Model file for the job. Use its own axes, mm. A direction names the side the tool comes from. Give positions to 0.01 mm unless a question says otherwise; leave off trailing zeros. Write each loop counter-clockwise with the first axis right and the second up, starting at its lowest first coordinate (ties: lowest second). Pieces come first, ordered by that corner, then holes. Notation, with made-up numbers: (79, 29.25) - (136, 29.25) arc R10 cw to (136, 44.25) - close; hole circle Ø6 at (7, 46). An arc over 180 degrees is marked (long way). Use CSV: the item, a comma, the result in double quotes.
from build123d import *

# Parameters (mm, degrees)
SKETCH1_W                 = 32.4
SKETCH1_H                 = 32.4
BOSS_EXTRUDE1_DEPTH       = 98.5
SKETCH2_R                 = 11.65
CUT_EXTRUDE1_DEPTH        = 88.5
SKETCH3_R                 = 6.5
CUT_EXTRUDE2_DEPTH        = 99.398410022
F_1_0MM_DOWEL_HOLE1_D     = 2.8
F_1_0MM_DOWEL_HOLE1_DEPTH = 7
F_1_0MM_DOWEL_HOLE1_TIP   = 0.841204867
SKETCH7_R                 = 2.5
CUT_EXTRUDE3_DEPTH        = 14
SKETCH8_W                 = 6.5
SKETCH8_H                 = 98.5
BOSS_EXTRUDE2_DEPTH       = 8.64
SKETCH14_W                = 30.956114244
SKETCH14_H                = 32.4
CUT_EXTRUDE6_DEPTH        = 50
SKETCH11_W                = 20.4
SKETCH11_H                = 31.75
CUT_EXTRUDE4_DEPTH        = 107.197037106
SKETCH12_W                = 20.4
SKETCH12_H                = 31.75
CUT_EXTRUDE5_DEPTH        = 15
SKETCH23_W                = 8.64
SKETCH23_H                = 6.5
BOSS_EXTRUDE3_DEPTH       = 11.5
F_1_0MM_DOWEL_HOLE3_D     = 2.8
F_1_0MM_DOWEL_HOLE3_DEPTH = 5
F_1_0MM_DOWEL_HOLE3_TIP   = 0.841204867


with BuildPart() as part:
    # Sketch1 → Boss-Extrude1 (new body)
    with BuildSketch(Plane(origin=(0, 0, 0), x_dir=(1, 0, 0), z_dir=(0, 1, 0))):
        with Locations((-6.730344165, -20.189509634)):
            Rectangle(SKETCH1_W, SKETCH1_H)
        Polygon((11.469655835, -27.889509634), (9.469655835, -29.389509634), (9.469655835, -31.389509634), (11.469655835, -32.889509634), align=None)
        Polygon((11.469655835, -7.489509634), (9.469655835, -8.989509634), (9.469655835, -10.989509634), (11.469655835, -12.489509634), align=None)
    extrude(amount=BOSS_EXTRUDE1_DEPTH)

    # Sketch2 → Cut-Extrude1 (cut)
    with BuildSketch(Plane(origin=(0, 98.5, 0), x_dir=(1, 0, 0), z_dir=(0, 1, 0))):
        with Locations(Location((-6.730344165, -20.189509634, 0), (0, 0, 270))):
            Circle(SKETCH2_R)
    extrude(amount=-CUT_EXTRUDE1_DEPTH, mode=Mode.SUBTRACT)

    # Sketch3 → Cut-Extrude2 (cut, through all)
    with BuildSketch(Plane(origin=(0, 10, 0), x_dir=(1, 0, 0), z_dir=(0, 1, 0))):
        with Locations(Location((-6.730344165, -20.189509634, 0), (0, 0, 270))):
            Circle(SKETCH3_R)
    extrude(amount=-CUT_EXTRUDE2_DEPTH, mode=Mode.SUBTRACT)

    # Ø1.0mm Dowel Hole1
    with Locations(Plane(origin=(0, 98.5, 0), x_dir=(1, 0, 0), z_dir=(0, 1, 0))):
        with Locations((-18.730344165, -8.189509634), (5.269655835, -8.189509634), (5.269655835, -32.189509634), (-18.730344165, -32.189509634)):
            Hole(F_1_0MM_DOWEL_HOLE1_D / 2, depth=F_1_0MM_DOWEL_HOLE1_DEPTH)
            with Locations((0, 0, -(F_1_0MM_DOWEL_HOLE1_DEPTH + F_1_0MM_DOWEL_HOLE1_TIP / 2))):  # 118° drill point
                Cone(0, F_1_0MM_DOWEL_HOLE1_D / 2, F_1_0MM_DOWEL_HOLE1_TIP, mode=Mode.SUBTRACT)

    # Sketch7 → Cut-Extrude3 (cut)
    with BuildSketch(Plane(origin=(0, 0, 3.989509634), x_dir=(-1, 0, 0), z_dir=(0, 0, -1))):
        with Locations((6.730344165, 4.5)):
            Circle(SKETCH7_R)
    extrude(amount=-CUT_EXTRUDE3_DEPTH, mode=Mode.SUBTRACT)

    # Sketch8 → Boss-Extrude2 (add)
    with BuildSketch(Plane(origin=(9.469655835, 0, 0), x_dir=(0, 0, -1), z_dir=(1, 0, 0))):
        with Locations((-20.189509634, 49.25)):
            Rectangle(SKETCH8_W, SKETCH8_H)
    extrude(amount=BOSS_EXTRUDE2_DEPTH)

    # Sketch14 → Cut-Extrude6 (cut)
    with BuildSketch(Plane.XZ):
        with Locations((24.947712957, 20.189509634)):
            Rectangle(SKETCH14_W, SKETCH14_H)
    extrude(amount=-CUT_EXTRUDE6_DEPTH, mode=Mode.SUBTRACT)

    # Sketch11 → Cut-Extrude4 (cut, through all)
    with BuildSketch(Plane.XY.offset(36.389509634)):
        with Locations((-6.730344165, 72.625)):
            Rectangle(SKETCH11_W, SKETCH11_H)
        with Locations((-6.730344165, 30.875)):
            Rectangle(SKETCH11_W, SKETCH11_H)
    extrude(amount=-CUT_EXTRUDE4_DEPTH, mode=Mode.SUBTRACT)

    # Sketch12 → Cut-Extrude5 (cut)
    with BuildSketch(Plane.ZY.offset(22.930344165)):
        with Locations((20.189509634, 72.625)):
            Rectangle(SKETCH12_W, SKETCH12_H)
        with Locations((20.189509634, 30.875)):
            Rectangle(SKETCH12_W, SKETCH12_H)
    extrude(amount=-CUT_EXTRUDE5_DEPTH, mode=Mode.SUBTRACT)

    # Sketch23 → Boss-Extrude3 (add)
    with BuildSketch(Plane(origin=(0, 98.5, 0), x_dir=(1, 0, 0), z_dir=(0, 1, 0))):
        with Locations((13.789655835, -20.189509634)):
            Rectangle(SKETCH23_W, SKETCH23_H)
    extrude(amount=BOSS_EXTRUDE3_DEPTH)

    # Ø1.0mm Dowel Hole3
    with Locations(Plane(origin=(18.109655835, 0, 0), x_dir=(0, 0, -1), z_dir=(1, 0, 0))):
        with Locations((-20.189509634, 105), (-20.189509634, 55), (-20.189509634, 65), (-20.189509634, 95)):
            Hole(F_1_0MM_DOWEL_HOLE3_D / 2, depth=F_1_0MM_DOWEL_HOLE3_DEPTH)
            with Locations((0, 0, -(F_1_0MM_DOWEL_HOLE3_DEPTH + F_1_0MM_DOWEL_HOLE3_TIP / 2))):  # 118° drill point
                Cone(0, F_1_0MM_DOWEL_HOLE3_D / 2, F_1_0MM_DOWEL_HOLE3_TIP, mode=Mode.SUBTRACT)


solid = part.part
(1) Wall check: probe 1 along Y at (x, z) = (-5, 33.5); probe 2 along Z at (x, y) = (-18, 34); probe 3 along Z at (x, y) = (15.4, 65). Give the ranges that are in metal, low to high. Write a range as [from, to].
Checked values:
probe 1,"y = [0, 15], [46.75, 56.75], [88.5, 98.5]"
probe 2,"z = [3.99, 9.99], [30.39, 36.39]"
probe 3,"z = [16.94, 18.79], [21.59, 23.44]"
(2) 3-axis set-ups, long thin cutter, end or side, ignore diameter. For faces 5 (the face through (4.89, 64.29, 21.04)), 6 (the face through (-19, 56.75, 20)), 7 (the face through (9.47, 104, 20)), 8 (the face through (-20, 72, 30.39)), 9 (the face through (-16.93, 72, 33)): which of +Z, -Z, +X, -X, +Y, -Y reach the whole face in a straight line?
Checked values:
face 5,"+Y"
face 6,"none"
face 7,"+Z, -Z, -X, +Y"
face 8,"-X"
face 9,"+Z, -Z"
(3) Saw through at D-D, the plane y = 4.5. List the corners of the cut face in (x, z).
Checked values:
outline,"(-22.93, 3.99) - (-9.23, 3.99) - (-9.23, 14.19) arc R6.5 cw (long way) to (-4.23, 14.19) - (-4.23, 3.99) - (9.47, 3.99) - (9.47, 36.39) - (-22.93, 36.39) - close"
(4) Pull direction Z, two halves, no side cores. Call faces 1 (the face through (5.573, 94.951, 33.556)), 2 (the face through (18.11, 80, 20)), 3 (the face through (-7, 49, 36.39)), 4 (the face through (5.49, 90.8, 32.28)): released by +Z, released by -Z, zero draft, split by the parting line, or undercut.
Checked values:
face 1,"undercut"
face 2,"zero draft"
face 3,"released by +Z"
face 4,"undercut"
(5) Saw through at A-A, the plane y = 45.5. List the corners of the cut face in (x, z).
Checked values:
outline,"(-22.93, 3.99) - (-16.93, 3.99) - (-16.93, 9.99) - (-22.93, 9.99) - close; (-22.93, 30.39) - (-16.93, 30.39) - (-16.93, 36.39) - (-22.93, 36.39) - close; (3.47, 3.99) - (9.47, 3.99) - (9.47, 36.39) - (3.47, 36.39) - (3.47, 25.82) arc R11.65 cw to (3.47, 14.56) - close"
(6) Flat gauge pins, fed straight in: P1, Ø15, axis at x = -6.73, z = 20.19, coming from the +Y side; P2, Ø6, axis at y = 55.5, z = 12, coming from the +X side; P3, Ø4.5, axis at x = 5.27, z = 8.19, coming from the +Y side; P4, Ø1.5, axis at x = -9, z = 16, coming from the -Y side. Where does each tip first touch, or does it go through?
Checked values:
P1,"stops at y = 10"
P2,"stops at x = 11.47"
P3,"stops at y = 98.5"
P4,"passes through"
(7) Saw through at C-C, the plane x = -2.5. List the corners of the cut face in (y, z).
Checked values:
outline,"(0, 3.99) - (15, 3.99) - (15, 9.33) - (10, 9.33) - (10, 15.25) - (0, 15.25) - close; (0, 25.12) - (10, 25.12) - (10, 31.04) - (15, 31.04) - (15, 36.39) - (0, 36.39) - close; (46.75, 3.99) - (56.75, 3.99) - (56.75, 9.33) - (46.75, 9.33) - close; (46.75, 31.04) - (56.75, 31.04) - (56.75, 36.39) - (46.75, 36.39) - close; (88.5, 3.99) - (98.5, 3.99) - (98.5, 9.33) - (88.5, 9.33) - close; (88.5, 31.04) - (98.5, 31.04) - (98.5, 36.39) - (88.5, 36.39) - close"
(8) Saw through at B-B, the plane x = 15. List the corners of the cut face in (y, z).
Checked values:
outline,"(50, 16.94) - (110, 16.94) - (110, 23.44) - (50, 23.44) - close; hole circle Ø2.8 at (55, 20.19); hole circle Ø2.8 at (65, 20.19); hole circle Ø2.8 at (95, 20.19); hole circle Ø2.8 at (105, 20.19)"
